Source: CAD feature listing. Evaluate the final solid. Frame: model axes, mm. A direction names the side the tool comes from. Give positions to 0.01 mm unless a question says otherwise; leave off trailing zeros. Write each loop counter-clockwise with the first axis right and the second up, starting at its lowest first coordinate (ties: lowest second). Pieces come first, ordered by that corner, then holes. Notation, with made-up numbers: (66, 13) -> (93, 13) arc R16 ccw to (93, 36) -> close; hole circle Ø2 at (-9.5, -39). An arc over 180 degrees is marked (long way). Use one line per item in the form item = value. Start each with the question number.
(1) Draft query along Z for faces 1 (the face through (0, 10, 53)), 2 (the face through (0, 1.5, -12)), 3 (the face through (-30, 11, -50)), 4 (the face through (-35.5, 10, 1)). Return one class per face: pulls with the +Z half, pulls with the -Z half, needs draft (parallel to the pull), parting line crosses it, or undercut.
(2) Set-up query: faces 5 (the face through (0, 0, -13)), 6 (the face through (32, 1.5, 49)). Return all of +Z, -Z, +X, -X, +Y, -Y with unobstructed straight access to the full face (end or side cutting, diameter ignored); none if empty.
(3) First-contact query: P1, Ø1.8, axis at x = 32, z = 49.5, coming from the +Y side. Flat tip, straight axial feed; report the tip coordinate or a pass-through.
(4) Cut plane D-D, the plane z = 15.5. Output: boundary loops of the cut face in (x, y).
(5) Cut plane B-B, the plane y = 9. Output: boundary loops of the cut face in (x, z).
(6) Cut plane C-C, the plane z = 1.5. Output: boundary loops of the cut face in (x, y).
(7) Cut plane A-A, the plane x = 19. Output: boundary loops of the cut face in (y, z), and give its area (3 significant figures).
(8) Material intervals for line 1 along Z through (x, y) = (-32, 12.5); line 2 along X through (y, z) = (15.25, -49.5); line 3 along Z through (x, y) = (2.5, 13.5), sorted ascending. Write a range as from..to.
from build123d import *

# Parameters (mm, degrees)
SKETCH2_W                                  = 71
SKETCH2_H                                  = 106
BOSS_EXTRUDE1_DEPTH                        = 21
SHELL1_T                                   = -1.5
SKETCH3_W                                  = 30
SKETCH3_H                                  = 5.5
CUT_EXTRUDE1_DEPTH                         = 21
SKETCH4_R                                  = 1.5
BOSS_EXTRUDE2_DEPTH                        = 19.5
MIRROR1_AT_THE_SECOND_PLANE_COPY_1_SKETC_R = 1.5
MIRROR1_AT_THE_SECOND_PLANE_COPY_1_DEPTH   = 19.5
SKETCH5_W                                  = 48
SKETCH5_H                                  = 23
CUT_EXTRUDE2_DEPTH                         = 1.5


with BuildPart() as part:
    # Sketch2 → Boss-Extrude1 (new body)
    with BuildSketch(Plane(origin=(0, 0, 0), x_dir=(1, 0, 0), z_dir=(0, 1, 0))):
        Rectangle(SKETCH2_W, SKETCH2_H)
    extrude(amount=BOSS_EXTRUDE1_DEPTH)

    # Shell1
    shell1_openings = [part.faces().sort_by_distance(p)[0] for p in [
        (0, 21, 0),
    ]]
    offset(amount=SHELL1_T, openings=shell1_openings, kind=Kind.INTERSECTION)

    # Sketch3 → Cut-Extrude1 (cut)
    with BuildSketch(Plane.XY.offset(53)):
        with Locations((-13, 18.25)):
            Rectangle(SKETCH3_W, SKETCH3_H)
    extrude(amount=-CUT_EXTRUDE1_DEPTH, mode=Mode.SUBTRACT)

    # Sketch4 → Boss-Extrude2 (add)
    with BuildSketch(Plane(origin=(0, 1.5, 0), x_dir=(1, 0, 0), z_dir=(0, 1, 0))):
        with BuildLine():
            Line((-34, 51.5), (-30, 51.5))
            Line((-30, 51.5), (-30, 48))
            ThreePointArc((-30, 48), (-30.146446609, 47.646446609), (-30.5, 47.5))
            Line((-30.5, 47.5), (-34, 47.5))
            Line((-34, 47.5), (-34, 51.5))
        make_face()
        with Locations((-32, 49.5)):
            Circle(SKETCH4_R, mode=Mode.SUBTRACT)
    boss_extrude2 = extrude(amount=BOSS_EXTRUDE2_DEPTH)

    # Mirror1: Boss-Extrude2 across plane
    add(boss_extrude2.mirror(Plane.ZY))

    # Mirror1 at the second plane: Boss-Extrude2 across plane
    add(boss_extrude2.mirror(Plane(origin=(0, 0, 0), x_dir=(1, 0, 0), z_dir=(0, 0, -1))))

    # Mirror1 at the second plane copy 1 sketc → Mirror1 at the second plane copy 1 (add)
    with BuildSketch(Plane(origin=(0, 1.5, 0), x_dir=(-1, 0, 0), z_dir=(0, 1, 0))):
        with BuildLine():
            Line((-34, 51.5), (-30, 51.5))
            Line((-30, 51.5), (-30, 48))
            ThreePointArc((-30, 48), (-30.146446609, 47.646446609), (-30.5, 47.5))
            Line((-30.5, 47.5), (-34, 47.5))
            Line((-34, 47.5), (-34, 51.5))
        make_face()
        with Locations((-32, 49.5)):
            Circle(MIRROR1_AT_THE_SECOND_PLANE_COPY_1_SKETC_R, mode=Mode.SUBTRACT)
    extrude(amount=MIRROR1_AT_THE_SECOND_PLANE_COPY_1_DEPTH)

    # Sketch5 → Cut-Extrude2 (cut)
    with BuildSketch(Plane(origin=(0, 1.5, 0), x_dir=(1, 0, 0), z_dir=(0, 1, 0))):
        Rectangle(SKETCH5_W, SKETCH5_H)
    extrude(amount=-CUT_EXTRUDE2_DEPTH, mode=Mode.SUBTRACT)


solid = part.part
Geometry says:
q1.face_1 = pulls with the +Z half
q1.face_2 = undercut
q1.face_3 = undercut
q1.face_4 = needs draft
q2.face_5 = +Z, -Z, +X, -X, -Y
q2.face_6 = +Y
q3.P1 = 1.5
q4.outline = (-35.5, 0) -> (35.5, 0) -> (35.5, 21) -> (34, 21) -> (34, 1.5) -> (-34, 1.5) -> (-34, 21) -> (-35.5, 21) -> close
q5.outline = (-35.5, -53) -> (35.5, -53) -> (35.5, 53) -> (-35.5, 53) -> close; hole (-34, -47.5) -> (-30.5, -47.5) arc R0.5 cw to (-30, -48) -> (-30, -51.5) -> (30, -51.5) -> (30, -48) arc R0.5 cw to (30.5, -47.5) -> (34, -47.5) -> (34, 47.5) -> (30.5, 47.5) arc R0.5 cw to (30, 48) -> (30, 51.5) -> (-30, 51.5) -> (-30, 48) arc R0.5 cw to (-30.5, 47.5) -> (-34, 47.5) -> close; hole circle Ø3 at (-32, -49.5); hole circle Ø3 at (-32, 49.5); hole circle Ø3 at (32, -49.5); hole circle Ø3 at (32, 49.5)
q6.outline = (-35.5, 0) -> (-24, 0) -> (-24, 1.5) -> (-34, 1.5) -> (-34, 21) -> (-35.5, 21) -> close; (24, 0) -> (35.5, 0) -> (35.5, 21) -> (34, 21) -> (34, 1.5) -> (24, 1.5) -> close
q7.outline = (0, -53) -> (21, -53) -> (21, -51.5) -> (1.5, -51.5) -> (1.5, -11.5) -> (0, -11.5) -> close; (0, 11.5) -> (1.5, 11.5) -> (1.5, 51.5) -> (21, 51.5) -> (21, 53) -> (0, 53) -> close
q7.area = 183 mm^2
q8.line_1 = -53..-51, -48..-47.5, 47.5..48, 51..53
q8.line_2 = -35.5..-33.5, -30.5..-30, 30..30.5, 33.5..35.5
q8.line_3 = -53..-51.5, 51.5..53
